Here's how the part is built. I have some questions about the finished solid (model axes, mm). Coordinates: 2 decimals unless noted, no trailing zeros.
from build123d import *

# Parameters (mm, degrees)
SKETCH1_R           = 2.6035
BOSS_EXTRUDE1_DEPTH = 279.4


with BuildPart() as part:
    # Sketch1 → Boss-Extrude1 (new body)
    with BuildSketch(Plane.XY):
        with BuildLine():
            Line((10.5918, 12.7), (10.5664, 12.7))
            ThreePointArc((10.5664, 12.7), (10.0584, 12.192), (9.5504, 12.7))
            Line((9.5504, 12.7), (6.3246, 12.7))
            ThreePointArc((6.3246, 12.7), (5.8166, 12.192), (5.3086, 12.7))
            Line((5.3086, 12.7), (4.3561, 12.7))
            ThreePointArc((4.3561, 12.7), (3.2512, 11.5951), (4.3561, 10.4902))
            Line((4.3561, 10.4902), (6.370083786, 10.4902))
            ThreePointArc((6.370083786, 10.4902), (7.348856743, 9.836204819), (7.119204175, 8.681663397))
            Line((7.119204175, 8.681663397), (3.88464389, 5.447103113))
            ThreePointArc((3.88464389, 5.447103113), (2.854599758, 4.758849627), (1.63957986, 4.517167143))
            Line((1.63957986, 4.517167143), (-1.63957986, 4.517167143))
            ThreePointArc((-1.63957986, 4.517167143), (-2.854599758, 4.758849627), (-3.88464389, 5.447103113))
            Line((-3.88464389, 5.447103113), (-7.119204175, 8.681663397))
            ThreePointArc((-7.119204175, 8.681663397), (-7.348856743, 9.836204819), (-6.370083786, 10.4902))
            Line((-6.370083786, 10.4902), (-4.3561, 10.4902))
            ThreePointArc((-4.3561, 10.4902), (-3.2512, 11.5951), (-4.3561, 12.7))
            Line((-4.3561, 12.7), (-5.3086, 12.7))
            ThreePointArc((-5.3086, 12.7), (-5.8166, 12.192), (-6.3246, 12.7))
            Line((-6.3246, 12.7), (-9.5504, 12.7))
            ThreePointArc((-9.5504, 12.7), (-10.0584, 12.192), (-10.5664, 12.7))
            Line((-10.5664, 12.7), (-10.5918, 12.7))
            ThreePointArc((-10.5918, 12.7), (-12.082522516, 12.082522516), (-12.7, 10.5918))
            Line((-12.7, 10.5918), (-12.7, 10.5664))
            ThreePointArc((-12.7, 10.5664), (-12.192, 10.0584), (-12.7, 9.5504))
            Line((-12.7, 9.5504), (-12.7, 6.3246))
            ThreePointArc((-12.7, 6.3246), (-12.192, 5.8166), (-12.7, 5.3086))
            Line((-12.7, 5.3086), (-12.7, 4.3561))
            ThreePointArc((-12.7, 4.3561), (-11.5951, 3.2512), (-10.4902, 4.3561))
            Line((-10.4902, 4.3561), (-10.4902, 6.370083786))
            ThreePointArc((-10.4902, 6.370083786), (-9.836204819, 7.348856743), (-8.681663397, 7.119204175))
            Line((-8.681663397, 7.119204175), (-5.447103113, 3.88464389))
            ThreePointArc((-5.447103113, 3.88464389), (-4.758849627, 2.854599758), (-4.517167143, 1.63957986))
            Line((-4.517167143, 1.63957986), (-4.517167143, -1.63957986))
            ThreePointArc((-4.517167143, -1.63957986), (-4.758849627, -2.854599758), (-5.447103113, -3.88464389))
            Line((-5.447103113, -3.88464389), (-8.681663397, -7.119204175))
            ThreePointArc((-8.681663397, -7.119204175), (-9.836204819, -7.348856743), (-10.4902, -6.370083786))
            Line((-10.4902, -6.370083786), (-10.4902, -4.3561))
            ThreePointArc((-10.4902, -4.3561), (-11.5951, -3.2512), (-12.7, -4.3561))
            Line((-12.7, -4.3561), (-12.7, -5.3086))
            ThreePointArc((-12.7, -5.3086), (-12.192, -5.8166), (-12.7, -6.3246))
            Line((-12.7, -6.3246), (-12.7, -9.5504))
            ThreePointArc((-12.7, -9.5504), (-12.192, -10.0584), (-12.7, -10.5664))
            Line((-12.7, -10.5664), (-12.7, -10.5918))
            ThreePointArc((-12.7, -10.5918), (-12.082522516, -12.082522516), (-10.5918, -12.7))
            Line((-10.5918, -12.7), (-10.5664, -12.7))
            ThreePointArc((-10.5664, -12.7), (-10.0584, -12.192), (-9.5504, -12.7))
            Line((-9.5504, -12.7), (-6.3246, -12.7))
            ThreePointArc((-6.3246, -12.7), (-5.8166, -12.192), (-5.3086, -12.7))
            Line((-5.3086, -12.7), (-4.3561, -12.7))
            ThreePointArc((-4.3561, -12.7), (-3.2512, -11.5951), (-4.3561, -10.4902))
            Line((-4.3561, -10.4902), (-6.370083786, -10.4902))
            ThreePointArc((-6.370083786, -10.4902), (-7.348856743, -9.836204819), (-7.119204175, -8.681663397))
            Line((-7.119204175, -8.681663397), (-3.88464389, -5.447103113))
            ThreePointArc((-3.88464389, -5.447103113), (-2.854599758, -4.758849627), (-1.63957986, -4.517167143))
            Line((-1.63957986, -4.517167143), (1.63957986, -4.517167143))
            ThreePointArc((1.63957986, -4.517167143), (2.854599758, -4.758849627), (3.88464389, -5.447103113))
            Line((3.88464389, -5.447103113), (7.119204175, -8.681663397))
            ThreePointArc((7.119204175, -8.681663397), (7.348856743, -9.836204819), (6.370083786, -10.4902))
            Line((6.370083786, -10.4902), (4.3561, -10.4902))
            ThreePointArc((4.3561, -10.4902), (3.2512, -11.5951), (4.3561, -12.7))
            Line((4.3561, -12.7), (5.3086, -12.7))
            ThreePointArc((5.3086, -12.7), (5.8166, -12.192), (6.3246, -12.7))
            Line((6.3246, -12.7), (9.5504, -12.7))
            ThreePointArc((9.5504, -12.7), (10.0584, -12.192), (10.5664, -12.7))
            Line((10.5664, -12.7), (10.5918, -12.7))
            ThreePointArc((10.5918, -12.7), (12.082522516, -12.082522516), (12.7, -10.5918))
            Line((12.7, -10.5918), (12.7, -10.5664))
            ThreePointArc((12.7, -10.5664), (12.192, -10.0584), (12.7, -9.5504))
            Line((12.7, -9.5504), (12.7, -6.3246))
            ThreePointArc((12.7, -6.3246), (12.192, -5.8166), (12.7, -5.3086))
            Line((12.7, -5.3086), (12.7, -4.3561))
            ThreePointArc((12.7, -4.3561), (11.5951, -3.2512), (10.4902, -4.3561))
            Line((10.4902, -4.3561), (10.4902, -6.370083786))
            ThreePointArc((10.4902, -6.370083786), (9.836204819, -7.348856743), (8.681663397, -7.119204175))
            Line((8.681663397, -7.119204175), (5.447103113, -3.88464389))
            ThreePointArc((5.447103113, -3.88464389), (4.758849627, -2.854599758), (4.517167143, -1.63957986))
            Line((4.517167143, -1.63957986), (4.517167143, 1.63957986))
            ThreePointArc((4.517167143, 1.63957986), (4.758849627, 2.854599758), (5.447103113, 3.88464389))
            Line((5.447103113, 3.88464389), (8.681663397, 7.119204175))
            ThreePointArc((8.681663397, 7.119204175), (9.836204819, 7.348856743), (10.4902, 6.370083786))
            Line((10.4902, 6.370083786), (10.4902, 4.3561))
            ThreePointArc((10.4902, 4.3561), (11.5951, 3.2512), (12.7, 4.3561))
            Line((12.7, 4.3561), (12.7, 5.3086))
            ThreePointArc((12.7, 5.3086), (12.192, 5.8166), (12.7, 6.3246))
            Line((12.7, 6.3246), (12.7, 9.5504))
            ThreePointArc((12.7, 9.5504), (12.192, 10.0584), (12.7, 10.5664))
            Line((12.7, 10.5664), (12.7, 10.5918))
            ThreePointArc((12.7, 10.5918), (12.082522516, 12.082522516), (10.5918, 12.7))
        make_face()
        Circle(SKETCH1_R, mode=Mode.SUBTRACT)
    extrude(amount=BOSS_EXTRUDE1_DEPTH)


solid = part.part
1. For pin 1 Ø1.6 at (x, z) = (0, 75) entering from +Y; pin 2 Ø12 at (x, z) = (-6, 174) entering from -Y; pin 3 Ø1 at (y, z) = (-0.5, 173.5) entering from +X; pin 4 Ø2.5 at (x, z) = (1, 72) entering from -Y, each with a flat end and sliding along its axis, tell me the tip position at first contact or that it passes through.
2. If I drill on line 1 (Y direction, x = 0, z = 210.5); line 2 (X direction, y = 2, z = 264); line 3 (Y direction, x = -5, z = 188.5), over which ranges is the centre line in solid material (lowest first)?
3. Thinking about a two-plate mould opening in X: for faces 1 (the face through (0, 3, 0)), 2 (the face through (2.483, 0.782, 137.744)), which applies, pulls with the +X half, pulls with the -X half, needs draft (parallel to the pull), parting line crosses it, or undercut?
Response values:
1. pin 1: stops at y = 4.52
1. pin 2: stops at y = -12.7
1. pin 3: stops at x = 4.52
1. pin 4: stops at y = -4.58
2. line 1: y = -4.52 to -2.6, 2.6 to 4.52
2. line 2: x = -4.54 to -1.67, 1.67 to 4.54
2. line 3: y = -12.7 to -10.49, -6.56 to -3.32, 3.32 to 6.56, 10.49 to 12.7
3. face 1: needs draft
3. face 2: undercut
